from build123d import *

# Parameters (mm, degrees)
SKETCH1_W               = 78.778264774
SKETCH1_H               = 80
BOSS_EXTRUDE1_DEPTH     = 45
SKETCH2_W               = 20.2
SKETCH2_H               = 20.2
CUT_EXTRUDE1_DEPTH      = 20
CUT_EXTRUDE2_DEPTH      = 1226.691607852
CUT_EXTRUDE2_DEPTH_BACK = 1226.691607852
SKETCH4_W               = 78.778264774
SKETCH4_H               = 80
BOSS_EXTRUDE2_DEPTH     = 56
CUT_EXTRUDE3_START      = -50.519806
SKETCH5_R               = 10
CUT_EXTRUDE3_DEPTH      = 50.519818
SKETCH6_R               = 3.4
BOSS_EXTRUDE3_DEPTH     = 12
SKETCH7_R               = 10
BOSS_EXTRUDE4_DEPTH     = 5
SKETCH8_R               = 3.4
BOSS_EXTRUDE5_DEPTH     = 1.5
SKETCH9_R               = 10
BOSS_EXTRUDE6_DEPTH     = 13.769806202
SKETCH10_W              = 31.75
SKETCH10_H              = 20
CUT_EXTRUDE4_DEPTH      = 41
SKETCH13_W              = 30.362291711
SKETCH13_H              = 20
CUT_EXTRUDE5_DEPTH      = 31.75
SKETCH11_R              = 3.4
BOSS_EXTRUDE7_DEPTH     = 14
SKETCH12_R              = 3.4
BOSS_EXTRUDE8_DEPTH     = 1.5
CUT_EXTRUDE6_DEPTH      = 1382.374333236
CUT_EXTRUDE6_DEPTH_BACK = 1382.374333236
SKETCH14_R              = 2.5
CUT_EXTRUDE7_DEPTH      = 1384.878879614
CUT_EXTRUDE7_DEPTH_BACK = 10
SKETCH15_R              = 6
CUT_EXTRUDE8_DEPTH      = 45
SKETCH17_R              = 3
CUT_EXTRUDE9_DEPTH      = 45
SKETCH18_W              = 13
SKETCH18_H              = 15
CUT_EXTRUDE10_DEPTH     = 21
SKETCH19_W              = 13
SKETCH19_H              = 15
CUT_EXTRUDE11_DEPTH     = 21
CHAMFER1_SIZE           = 3
SKETCH20_R              = 5.5
CUT_EXTRUDE12_DEPTH     = 8
CUT_EXTRUDE13_START     = -8
SKETCH21_R              = 5.5
CUT_EXTRUDE13_DEPTH     = 8


with BuildPart() as part:
    # Sketch1 → Boss-Extrude1 (new body)
    with BuildSketch(Plane.YZ):
        with Locations((-601.571748543, 1182.329293832)):
            Rectangle(SKETCH1_W, SKETCH1_H)
    extrude(amount=BOSS_EXTRUDE1_DEPTH)

    # Sketch2 → Cut-Extrude1 (cut)
    with BuildSketch(Plane.XY.offset(1222.329293832)):
        with Locations((10.1, -579.082515944)):
            Rectangle(SKETCH2_W, SKETCH2_H)
    extrude(amount=-CUT_EXTRUDE1_DEPTH, mode=Mode.SUBTRACT)

    # Sketch3 → Cut-Extrude2 (cut, two sides: drawn at the far end of the back side and taken through both)
    with BuildSketch(Plane(origin=(0, -562.182616156, 0), x_dir=(-1, 0, 0), z_dir=(0, 1, 0)).offset(-CUT_EXTRUDE2_DEPTH_BACK)):
        with BuildLine():
            ThreePointArc((-11.102244776, 1215.119465234), (-13, 1212.329293832), (-11.102244776, 1209.53912243))
            Line((-11.102244776, 1209.53912243), (-11.102244776, 1215.119465234))
        make_face()
        with BuildLine():
            Line((-11.102244776, 1215.119465234), (-11.102244776, 1209.53912243))
            ThreePointArc((-11.102244776, 1209.53912243), (-10, 1209.329293832), (-8.897755224, 1209.53912243))
            Line((-8.897755224, 1209.53912243), (-8.897755224, 1215.119465234))
            ThreePointArc((-8.897755224, 1215.119465234), (-10, 1215.329293832), (-11.102244776, 1215.119465234))
        make_face()
        with BuildLine():
            Line((-8.897755224, 1215.119465234), (-8.897755224, 1209.53912243))
            ThreePointArc((-8.897755224, 1209.53912243), (-7.519401853, 1210.642097093), (-7, 1212.329293832))
            ThreePointArc((-7, 1212.329293832), (-7.519401853, 1214.016490571), (-8.897755224, 1215.119465234))
        make_face()
    extrude(amount=CUT_EXTRUDE2_DEPTH + CUT_EXTRUDE2_DEPTH_BACK, mode=Mode.SUBTRACT)

    # Sketch4 → Boss-Extrude2 (add)
    with BuildSketch(Plane.YZ.offset(45)):
        with Locations((-601.571748543, 1182.329293832)):
            Rectangle(SKETCH4_W, SKETCH4_H)
    extrude(amount=BOSS_EXTRUDE2_DEPTH)

    # Sketch5 → Cut-Extrude3 (cut)
    with BuildSketch(Plane.YZ.offset(101).offset(CUT_EXTRUDE3_START)):
        with Locations(Location((-592.544907867, 1182.329293832, 0), (0, 0, 270))):
            Circle(SKETCH5_R)
    extrude(amount=CUT_EXTRUDE3_DEPTH, mode=Mode.SUBTRACT)

    # Sketch6 → Boss-Extrude3 (add)
    with BuildSketch(Plane(origin=(57.230193798, 0, 0), x_dir=(0, -1, 0), z_dir=(-1, 0, 0))):
        with Locations(Location((592.544907867, 1182.329293832, 0), (0, 0, 180))):
            Circle(SKETCH6_R)
    extrude(amount=BOSS_EXTRUDE3_DEPTH)

    # Sketch7 → Boss-Extrude4 (add)
    with BuildSketch(Plane.YZ.offset(50.480193798)):
        with Locations(Location((-592.544907867, 1182.329293832, 0), (0, 0, 270))):
            Circle(SKETCH7_R)
    extrude(amount=BOSS_EXTRUDE4_DEPTH)



with BuildPart() as body_2:
    # Sketch8 → Boss-Extrude5 (new body)
    with BuildSketch(Plane.YZ.offset(85.730193798)):
        with Locations((-592.544907867, 1182.329293832)):
            Circle(SKETCH8_R)
    extrude(amount=BOSS_EXTRUDE5_DEPTH)


with BuildPart() as part_1:
    add(part.part)

    add(body_2.part)  # Boss-Extrude6 merges body 2
    # Sketch9 → Boss-Extrude6 (add)
    with BuildSketch(Plane.YZ.offset(87.230193798)):
        with Locations((-592.544907867, 1182.329293832)):
            Circle(SKETCH9_R)
    extrude(amount=BOSS_EXTRUDE6_DEPTH)

    # Sketch10 → Cut-Extrude4 (cut)
    with BuildSketch(Plane.XY.offset(1222.329293832)):
        with Locations((71.355193798, -592.719907867)):
            Rectangle(SKETCH10_W, SKETCH10_H)
    extrude(amount=-CUT_EXTRUDE4_DEPTH, mode=Mode.SUBTRACT)

    # Sketch13 → Cut-Extrude5 (cut)
    with BuildSketch(Plane.YZ.offset(55.480193798)):
        with Locations((-577.363762012, 1182.329293832)):
            Rectangle(SKETCH13_W, SKETCH13_H)
    extrude(amount=CUT_EXTRUDE5_DEPTH, mode=Mode.SUBTRACT)

    # Sketch11 → Boss-Extrude7 (add)
    with BuildSketch(Plane.YZ.offset(57.230193798)):
        with Locations((-592.544907867, 1182.329293832)):
            Circle(SKETCH11_R)
    extrude(amount=-BOSS_EXTRUDE7_DEPTH)

    # Sketch12 → Boss-Extrude8 (add)
    with BuildSketch(Plane(origin=(85.730193798, 0, 0), x_dir=(0, -1, 0), z_dir=(-1, 0, 0))):
        with Locations(Location((592.544907867, 1182.329293832, 0), (0, 0, 180))):
            Circle(SKETCH12_R)
    extrude(amount=-BOSS_EXTRUDE8_DEPTH)

    # Sketch14 → Cut-Extrude6 (cut, two sides: drawn at the far end of the back side and taken through both)
    with BuildSketch(Plane.YZ.offset(57.230193798).offset(-CUT_EXTRUDE6_DEPTH_BACK)):
        with Locations((-592.544907867, 1182.329293832)):
            Circle(SKETCH14_R)
    extrude(amount=CUT_EXTRUDE6_DEPTH + CUT_EXTRUDE6_DEPTH_BACK, mode=Mode.SUBTRACT)

    # Sketch15 → Cut-Extrude7 (cut, two sides: drawn at the far end of the back side and taken through both)
    with BuildSketch(Plane.YZ.offset(101).offset(-CUT_EXTRUDE7_DEPTH_BACK)):
        with Locations(Location((-592.544907867, 1182.329293832, 0), (0, 0, 270))):
            Circle(SKETCH15_R)
    extrude(amount=CUT_EXTRUDE7_DEPTH + CUT_EXTRUDE7_DEPTH_BACK, mode=Mode.SUBTRACT)

    # Sketch16 → Cut-Extrude8 (cut)
    with BuildSketch(Plane(origin=(0, 0, 0), x_dir=(0, -1, 0), z_dir=(-1, 0, 0))):
        Polygon((589.946831656, 1177.829293832), (595.142984078, 1177.829293832), (597.74106029, 1182.329293832), (595.142984078, 1186.829293832), (589.946831656, 1186.829293832), (587.348755444, 1182.329293832), align=None)
    extrude(amount=-CUT_EXTRUDE8_DEPTH, mode=Mode.SUBTRACT)

    # Sketch17 → Cut-Extrude9 (cut)
    with BuildSketch(Plane(origin=(0, 0, 0), x_dir=(0, -1, 0), z_dir=(-1, 0, 0))):
        with Locations(Location((569.682616156, 1157.329293832, 0), (0, 0, 90))):
            Circle(SKETCH17_R)
        with Locations(Location((633.46088093, 1157.329293832, 0), (0, 0, 90))):
            Circle(SKETCH17_R)
        with Locations(Location((569.682616156, 1192.329293832, 0), (0, 0, 90))):
            Circle(SKETCH17_R)
        with Locations(Location((633.46088093, 1192.329293832, 0), (0, 0, 90))):
            Circle(SKETCH17_R)
    extrude(amount=-CUT_EXTRUDE9_DEPTH, mode=Mode.SUBTRACT)

    # Sketch18 → Cut-Extrude10 (cut)
    with BuildSketch(Plane(origin=(0, -562.182616156, 0), x_dir=(-1, 0, 0), z_dir=(0, 1, 0))):
        with Locations((-21.5, 1157.329293832)):
            Rectangle(SKETCH18_W, SKETCH18_H)
        with Locations((-21.5, 1192.329293832)):
            Rectangle(SKETCH18_W, SKETCH18_H)
    extrude(amount=-CUT_EXTRUDE10_DEPTH, mode=Mode.SUBTRACT)

    # Sketch19 → Cut-Extrude11 (cut)
    with BuildSketch(Plane.XZ.offset(640.96088093)):
        with Locations((21.5, 1157.329293832)):
            Rectangle(SKETCH19_W, SKETCH19_H)
        with Locations((21.5, 1192.329293832)):
            Rectangle(SKETCH19_W, SKETCH19_H)
    extrude(amount=-CUT_EXTRUDE11_DEPTH, mode=Mode.SUBTRACT)

    # Chamfer1
    chamfer1_edges = [part_1.edges().sort_by_distance(p)[0] for p in [
        (101, -601.571748543, 1222.329293832),
        (101, -640.96088093, 1182.329293832),
        (101, -601.571748543, 1142.329293832),
        (101, -562.182616156, 1182.329293832),
        (50.5, -640.96088093, 1222.329293832),
        (50.5, -562.182616156, 1222.329293832),
        (50.5, -562.182616156, 1142.329293832),
        (50.5, -640.96088093, 1142.329293832),
    ]]
    chamfer(chamfer1_edges, length=CHAMFER1_SIZE)

    # Sketch20 → Cut-Extrude12 (cut)
    with BuildSketch(Plane(origin=(0, -562.182616156, 0), x_dir=(-1, 0, 0), z_dir=(0, 1, 0))):
        with Locations(Location((-10, 1212.329293832, 0), (0, 0, 90))):
            Circle(SKETCH20_R)
    extrude(amount=-CUT_EXTRUDE12_DEPTH, mode=Mode.SUBTRACT)

    # Sketch21 → Cut-Extrude13 (cut)
    with BuildSketch(Plane.XZ.offset(640.96088093).offset(CUT_EXTRUDE13_START)):
        with Locations(Location((10, 1212.329293832, 0), (0, 0, 90))):
            Circle(SKETCH21_R)
    extrude(amount=CUT_EXTRUDE13_DEPTH, mode=Mode.SUBTRACT)


solid = part_1.part
The model under review builds one solid part; all positions refer to its coordinate system, in mm. A direction names the side the tool comes from. Coordinates: 2 decimals unless noted, no trailing zeros. Loops run counter-clockwise (first coordinate to the right, second up) from the corner with the lowest first, then second, coordinate; pieces in that order, holes last.
(1) Wall thickness on L1, parallel to X at y = -577, z = 1187; L2, parallel to Z at x = 67, y = -569; L3, parallel to X at y = -602.5, z = 1191.5: over which ranges is each line inside the solid? List them lowest first.
Determined:
L1: x = 0 to 15, 28 to 55.48, 87.23 to 101
L2: z = 1142.33 to 1172.33, 1192.33 to 1222.33
L3: x = 0 to 55.48, 87.23 to 101
(2) Consider section C-C, the plane y = -601. Give the boundary of the cut face in (x, z).
Determined:
outline: (0, 1142.33) - (98, 1142.33) - (101, 1145.33) - (101, 1219.33) - (98, 1222.33) - (87.23, 1222.33) - (87.23, 1176.99) - (55.48, 1176.99) - (55.48, 1222.33) - (0, 1222.33) - close; hole circle Ø6 at (10, 1212.33)
(3) Consider section B-B, the plane x = 93.5. Give the boundary of the cut face in (y, z), plus the area to 3 significant figures.
Determined:
outline: (-640.96, 1145.33) - (-637.96, 1142.33) - (-565.18, 1142.33) - (-562.18, 1145.33) - (-562.18, 1219.33) - (-565.18, 1222.33) - (-637.96, 1222.33) - (-640.96, 1219.33) - close; hole circle Ø12 at (-592.54, 1182.33)
area: 6,170 mm2
(4) Tool access review of faces 4 (the flat face through (71, -602.72, 1202)), 5 (the flat face through (21, -631, 1149.829)), 6 (the cylindrical face through (36.38, -570.83, 1195.1)): name each direction out of +Z, -Z, +X, -X, +Y, -Y from which nothing blocks a thin tool from reaching the whole face with its end or side.
Determined:
face 4: +Z
face 5: -Y
face 6: -X
(5) Draft analysis for pull direction Z (two halves, no side actions). For faces 1 (the flat face through (98.948, -639.107, 1220.235)), 2 (the cylindrical face through (86.47, -595.94, 1182.18)), 3 (the flat face through (85.73, -595, 1181)), state which applies: +Z half, -Z half, draft (parallel to the pull), parting line (faces both ways), or undercut.
Determined:
face 1: +Z half
face 2: undercut
face 3: draft
(6) Insertion check: P1, Ø7.5, axis at y = -592.5, z = 1182, coming from the +X side; P2, Ø3, axis at x = 64.5, y = -587.5, coming from the +Z side; P3, Ø5, axis at y = -569.68, z = 1192.33, coming from the -X side. Each pin has a flat end and moves straight along its axis. Give the tip position at first contact, or say it passes through.
Determined:
P1: stops at x = 91
P2: stops at z = 1172.33
P3: stops at x = 45
(7) Consider section A-A, the plane y = -581.5. Give the boundary of the cut face in (x, z).
Determined:
outline: (0, 1142.33) - (98, 1142.33) - (101, 1145.33) - (101, 1219.33) - (98, 1222.33) - (20.2, 1222.33) - (20.2, 1202.33) - (0, 1202.33) - close; hole (15, 1149.83) - (28, 1149.83) - (28, 1164.83) - (15, 1164.83) - close; hole (15, 1184.83) - (28, 1184.83) - (28, 1199.83) - (15, 1199.83) - close; hole (55.48, 1172.33) - (87.23, 1172.33) - (87.23, 1192.33) - (55.48, 1192.33) - close
